Geometry: final body of the model. Coordinates: model frame, mm. Face numbers are marked on the shaded views. A direction names the side the tool comes from. Coordinates: 2 decimals unless noted, no trailing zeros. Order: outer loops, then holes, each group sorted by start corner. A loop starts at its lowest first (then second) coordinate and runs counter-clockwise, first axis right, second up. Notation, with made-up numbers: (-23.5, 44) -> (-13.5, 44) arc R35 cw to (-13.5, 80) -> close; hole circle Ø7 at (81, -34.5). An arc over 180 degrees is marked (long way). Answer in a Markdown table with one row per item. Add a question column.
1) Set-up query: the marked faces 1 and 2. Return all of +Z, -Z, +X, -X, +Y, -Y with unobstructed straight access to the full face (end or side cutting, diameter ignored); none if empty.
2) Section query C-C on x = -1. Return the cut outline in (y, z), then the cut area to 3 significant figures.
3) Pull-direction query (Z, two-part tool) for the marked faces 3, 4 and 5; classes: +Z half, -Z half, draft (parallel to the pull), parting line (faces both ways), or undercut.
4) Ray query, line 1 (X direction, y = 5, z = -67); line 2 (Z direction, x = -15.5, y = 3); line 3 (X direction, y = 33, z = 6). Return the intervals inside material, ascending. Write a range as from..to.
5) Contact query for flat-ended pins moving along their axis: P1, Ø8, axis at x = 28.5, z = -64.5, coming from the +Y side; P2, Ø8, axis at y = 19, z = 28, coming from the +X side; P3, Ø1.5, axis at x = -21, y = 16, coming from the -Z side; P4, Ø4.5, axis at x = 29.5, z = -67, coming from the -Y side. Output: stop coordinate, or through.
6) Section query A-A on x = -29.5. Count the separate pieces of the cut face and the enclosed holes in it, then the cut area to 3 significant figures.
7) Section query D-D on y = 20.5. Return the cut outline in (x, z).
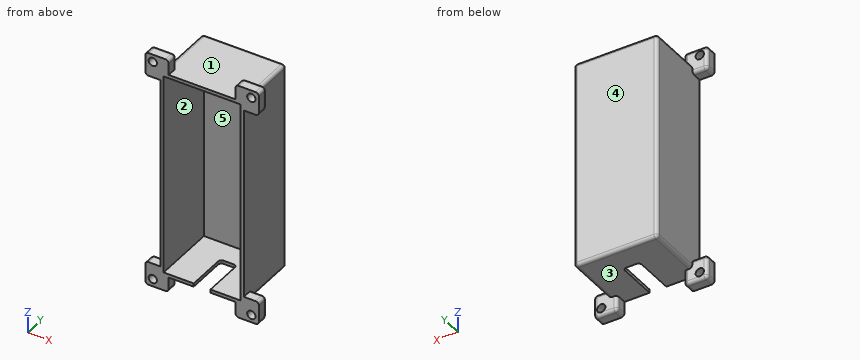
```python
from build123d import *

# Parameters (mm, degrees)
SKETCH1_W                                  = 50
SKETCH1_H                                  = 125
BOSS_EXTRUDE1_DEPTH                        = 40
SHELL2_T                                   = -2
SKETCH3_R                                  = 2.5
BOSS_EXTRUDE2_DEPTH                        = 7
MIRROR2_AT_THE_SECOND_PLANE_COPY_1_SKETC_R = 2.5
MIRROR2_AT_THE_SECOND_PLANE_COPY_1_DEPTH   = 7
CUT_EXTRUDE1_REACH                         = 145.917
SKETCH4_W                                  = 10
SKETCH4_H                                  = 25
FILLET2_R                                  = 2
FILLET3_R                                  = 2


with BuildPart() as part:
    # Sketch1 → Boss-Extrude1 (new body)
    with BuildSketch(Plane(origin=(0, 0, 0), x_dir=(1, 0, 0), z_dir=(0, 1, 0))):
        Rectangle(SKETCH1_W, SKETCH1_H)
    extrude(amount=BOSS_EXTRUDE1_DEPTH)

    # Shell2
    shell2_openings = [part.faces().sort_by_distance(p)[0] for p in [
        (0, 0, 0),
    ]]
    offset(amount=SHELL2_T, openings=shell2_openings, kind=Kind.INTERSECTION)

    # Sketch3 → Boss-Extrude2 (add)
    with BuildSketch(Plane(origin=(0, 0, 0), x_dir=(1, 0, 0), z_dir=(0, 1, 0))):
        Polygon((25, -62.5), (20, -62.5), (20, -71.5), (34, -71.5), (34, -57.5), (25, -57.5), align=None)
        with Locations(Location((29.5, -67, 0), (0, 0, 270))):
            Circle(SKETCH3_R, mode=Mode.SUBTRACT)
    boss_extrude2 = extrude(amount=BOSS_EXTRUDE2_DEPTH)

    # Mirror2: Boss-Extrude2 across plane
    add(boss_extrude2.mirror(Plane.XY))

    # Mirror2 at the second plane: Boss-Extrude2 across plane
    add(boss_extrude2.mirror(Plane(origin=(0, 0, 0), x_dir=(0, 0, 1), z_dir=(1, 0, 0))))

    # Mirror2 at the second plane copy 1 sketc → Mirror2 at the second plane copy 1 (add)
    with BuildSketch(Plane(origin=(0, 0, 0), x_dir=(-1, 0, 0), z_dir=(0, 1, 0))):
        Polygon((25, -62.5), (20, -62.5), (20, -71.5), (34, -71.5), (34, -57.5), (25, -57.5), align=None)
        with Locations(Location((29.5, -67, 0), (0, 0, 270))):
            Circle(MIRROR2_AT_THE_SECOND_PLANE_COPY_1_SKETC_R, mode=Mode.SUBTRACT)
    extrude(amount=MIRROR2_AT_THE_SECOND_PLANE_COPY_1_DEPTH)

    # Sketch4 → Cut-Extrude1 (cut, up to next)
    with BuildSketch(Plane(origin=(0, 0, -62.5), x_dir=(-1, 0, 0), z_dir=(0, 0, -1)), mode=Mode.PRIVATE) as cut_extrude1_sk1:
        with Locations((0, 12.5)):
            Rectangle(SKETCH4_W, SKETCH4_H)
    cut_extrude1_tool1 = extrude(cut_extrude1_sk1.sketch, amount=-CUT_EXTRUDE1_REACH, mode=Mode.PRIVATE) & part.part
    add(cut_extrude1_tool1.solids().sort_by_distance((0, 12.5, -62.5))[0], mode=Mode.SUBTRACT)

    # Fillet2
    fillet2_edges = [part.edges().sort_by_distance(p)[0] for p in [
        (-25, 40, 0),
        (0, 40, 62.5),
        (20, 7, 67),
        (27, 7, 71.5),
        (34, 7, 64.5),
        (29.5, 7, 57.5),
        (20, 3.5, 71.5),
        (34, 3.5, 71.5),
        (34, 3.5, 57.5),
        (-29.5, 7, 57.5),
        (-34, 7, 64.5),
        (-34, 3.5, 57.5),
        (25, 40, 0),
        (-27, 7, 71.5),
        (-34, 3.5, 71.5),
        (-20, 7, 67),
        (-20, 3.5, 71.5),
        (29.5, 7, -57.5),
        (34, 7, -64.5),
        (34, 3.5, -57.5),
        (27, 7, -71.5),
        (34, 3.5, -71.5),
        (20, 7, -67),
        (20, 3.5, -71.5),
        (25, 23.5, 62.5),
        (-25, 23.5, 62.5),
        (-25, 23.5, -62.5),
        (25, 23.5, -62.5),
        (-20, 7, -67),
        (-27, 7, -71.5),
        (-34, 7, -64.5),
        (-29.5, 7, -57.5),
        (-20, 3.5, -71.5),
        (-34, 3.5, -71.5),
        (-34, 3.5, -57.5),
        (0, 40, -62.5),
    ]]
    fillet(fillet2_edges, radius=FILLET2_R - 0.0001)  # a hair under: the kernel refuses the full size

    # Fillet3
    fillet3_edges = [part.edges().sort_by_distance(p)[0] for p in [
        (5, 25, -61.5),
        (-5, 25, -61.5),
    ]]
    fillet(fillet3_edges, radius=FILLET3_R)


solid = part.part
```
Result:
| question | item | result |
|---|---|---|
| 1 | face 1 | +Z, +Y |
| 1 | face 2 | -Y |
| 2 | outline | (0, 60.5) -> (38, 60.5) -> (38, -60.5) -> (25, -60.5) -> (25, -62.5) -> (38, -62.5) arc R2 ccw to (40, -60.5) -> (40, 60.5) arc R2 ccw to (38, 62.5) -> (0, 62.5) -> close |
| 2 | area | 350 mm2 |
| 3 | face 3 | -Z half |
| 3 | face 4 | draft |
| 3 | face 5 | undercut |
| 4 | line 1 | -34..-32, -27..-20, 20..27, 32..34 |
| 4 | line 2 | -62.5..-60.5, 60.5..62.5 |
| 4 | line 3 | -25..-23, 23..25 |
| 5 | P1 | y = 7 |
| 5 | P2 | x = 25 |
| 5 | P3 | z = -62.5 |
| 5 | P4 | through |
| 6 | separate pieces | 4 |
| 6 | enclosed holes | 0 |
| 6 | area | 123 mm2 |
| 7 | outline | (-25, -60.5) arc R2 ccw to (-23, -62.5) -> (-5, -62.5) -> (-5, -60.5) -> (-23, -60.5) -> (-23, 60.5) -> (23, 60.5) -> (23, -60.5) -> (5, -60.5) -> (5, -62.5) -> (23, -62.5) arc R2 ccw to (25, -60.5) -> (25, 60.5) arc R2 ccw to (23, 62.5) -> (-23, 62.5) arc R2 ccw to (-25, 60.5) -> close |
